from build123d import *

# Parameters (mm, degrees)
F1_DEPTH      = 3.175
F2_R          = 1.524
F5_START      = -3.175
F4_R          = 19.05
F5_DEPTH      = 66.675
F3_R          = 12.7
F6_DEPTH      = 63.5
F6_DEPTH_BACK = 25.4
F7_R          = 4.7625
F8_DEPTH      = 75.09229


with BuildPart() as f1:
    # F0 (on Top) → F1 (new body, symmetric)
    with BuildSketch(Plane.XY):
        with BuildLine():
            Line((52.7649549718, 29.4761320562), (-48.8350450282, 29.4761320562))
            Line((-48.8350450282, 29.4761320562), (-48.8350450282, 20.0781320562))
            Line((-48.8350450282, 20.0781320562), (-26.1262064392, 20.0781320562))
            ThreePointArc((-26.1262064392, 20.0781320562), (-16.4742064392, 10.4261320562), (-26.1262064392, 0.7741320562))
            Line((-26.1262064392, 0.7741320562), (-48.8350450282, 0.7741320562))
            Line((-48.8350450282, 0.7741320562), (-48.8350450282, -8.6238679438))
            Line((-48.8350450282, -8.6238679438), (52.7649549718, -8.6238679438))
            Line((52.7649549718, -8.6238679438), (52.7649549718, 0.7741320562))
            Line((52.7649549718, 0.7741320562), (30.0561163827, 0.7741320562))
            ThreePointArc((30.0561163827, 0.7741320562), (20.4041163827, 10.4261320562), (30.0561163827, 20.0781320562))
            Line((30.0561163827, 20.0781320562), (52.7649549718, 20.0781320562))
            Line((52.7649549718, 20.0781320562), (52.7649549718, 29.4761320562))
        make_face()
    extrude(amount=F1_DEPTH, both=True)

    # F2
    f2_edges = [f1.edges().sort_by_distance(p)[0] for p in [
        (52.764955, 29.476132, 0),
        (52.764955, -8.623868, 0),
        (-48.835045, -8.623868, 0),
        (-48.835045, 29.476132, 0),
    ]]
    fillet(f2_edges, radius=F2_R)

    # F4 (on Top) → F5 (join)
    with BuildSketch(Plane.XY.offset(F5_START)):
        with Locations((1.9649549718, 10.4261320562)):
            Circle(F4_R)
    extrude(amount=-F5_DEPTH)

    # F3 (on Top) → F6 (cut, two sides)
    with BuildSketch(Plane.XY) as f6_sk:
        with Locations((1.9649549718, 10.4261320562)):
            Circle(F3_R)
    extrude(amount=-F6_DEPTH, mode=Mode.SUBTRACT)
    extrude(f6_sk.sketch, amount=F6_DEPTH_BACK, mode=Mode.SUBTRACT)

    # F7 (on Top) → F8 (cut)
    with BuildSketch(Plane.XY):
        with Locations((1.9649549718, 10.4261320562)):
            Circle(F7_R)
    extrude(amount=-F8_DEPTH, mode=Mode.SUBTRACT)


solid = f1.part
Input: part model. Units: mm. Frame: model coordinates. A direction names the side the tool comes from. Coordinates: 2 decimals unless noted, no trailing zeros. Loops run counter-clockwise (first coordinate to the right, second up) from the corner with the lowest first, then second, coordinate; pieces in that order, holes last.
Q1. Draft query along X for faces 1 (the face through (20.406, 10.214, 0.044)), 2 (the face through (-13.15, -1.17, -36.05)), 3 (the face through (0.933, 5.777, -66.631)), 4 (the face through (-37, 0.774, 0)). Return one class per face: +X half, -X half, draft (parallel to the pull), parting line (faces both ways), or undercut.
Q2. Contact query for flat-ended pins moving along their axis: pin 1 (1.5 mm diameter, centred on x = -23, y = 20, fed in from -Z) (3 decimals); pin 2 (1.5 mm diameter, centred on x = -30.5, y = 18, fed in from +Z); pin 3 (1 mm diameter, centred on y = 14.5, z = -47.5, fed in from -X); pin 4 (1.5 mm diameter, centred on y = 22, z = -61.5, fed in from -X). Output: stop coordinate, or through.
Q3. Material intervals for line 1 (Z direction, x = 25.5, y = 0.5) (3 decimals); line 2 (Y direction, x = -5.5, z = -25); line 3 (X direction, y = 4, z = -13), sorted ascending.
Q4. Cut plane A-A (x = -38). Output: boundary loops of the cut face in (y, z) (3 decimals).
Q5. Cut plane C-C (x = 16.5). Output: boundary loops of the cut face in (y, z) (3 decimals).
Q6. Cut plane B-B (y = 19). Output: boundary loops of the cut face in (x, z) (3 decimals).
Q7. Set-up query: faces 5 (the face through (-38, 20.078, 0)), 6 (the face through (-0.79, -1.97, -30.63)), 7 (the face through (52.765, 24, 0)), 8 (the face through (42, 0.774, 0)), 9 (the face through (-29, -4, -3.175)). Return all of +Z, -Z, +X, -X, +Y, -Y with unobstructed straight access to the full face (end or side cutting, diameter ignored); none if empty.
Q8. Cut plane D-D (z = -26.5). Output: boundary loops of the cut face in (x, y), then the cut area to 3 significant figures.
Working result:
1. face 1: +X half
1. face 2: parting line
1. face 3: undercut
1. face 4: draft
2. pin 1: stops at z = -3.175
2. pin 2: passes through
2. pin 3: stops at x = -16.75
2. pin 4: stops at x = -13.71
3. line 1: z = -3.175 to 3.175
3. line 2: y = -7.1 to 0.15, 20.7 to 27.95
3. line 3: x = -15.97 to -8.99, 12.92 to 19.9
4. outline: (-8.624, -3.175) - (0.774, -3.175) - (0.774, 3.175) - (-8.624, 3.175) - close; (20.078, -3.175) - (29.476, -3.175) - (29.476, 3.175) - (20.078, 3.175) - close
5. outline: (-8.624, -3.175) - (-1.888, -3.175) - (-1.888, -69.85) - (22.74, -69.85) - (22.74, -3.175) - (29.476, -3.175) - (29.476, 3.175) - (-8.624, 3.175) - close
6. outline: (-21.693, -3.175) - (-15.047, -3.175) - (-15.047, -69.85) - (18.976, -69.85) - (18.976, -3.175) - (25.623, -3.175) - (25.623, 3.175) - (11.334, 3.175) - (11.334, -63.5) - (-7.404, -63.5) - (-7.404, 3.175) - (-21.693, 3.175) - close
7. face 5: +Z, -Z, -X
7. face 6: +Z
7. face 7: +Z, -Z, +X, +Y, -Y
7. face 8: +Z, -Z, +X
7. face 9: -Z, -X, -Y
8. outline: circle Ø38.1 at (1.96, 10.43); hole circle Ø25.4 at (1.96, 10.43)
8. area: 633 mm2
